```python
from build123d import *

# Parameters (mm, degrees)
SKETCH1_R               = 15.5
BOSS_EXTRUDE1_DEPTH     = 5
CUT_EXTRUDE1_REACH      = 24.483
SKETCH2_R               = 3
CUT_EXTRUDE2_DEPTH      = 23.483327156
CUT_EXTRUDE2_DEPTH_BACK = 23.483327156
SKETCH3_R               = 1.525


with BuildPart() as part:
    # Sketch1 → Boss-Extrude1 (new body)
    with BuildSketch(Plane.XY):
        Circle(SKETCH1_R)
    extrude(amount=BOSS_EXTRUDE1_DEPTH)

    # Sketch2 → Cut-Extrude1 (cut, up to next)
    with BuildSketch(Plane.XY.offset(5), mode=Mode.PRIVATE) as cut_extrude1_sk1:
        Circle(SKETCH2_R)
    cut_extrude1_tool1 = extrude(cut_extrude1_sk1.sketch, amount=-CUT_EXTRUDE1_REACH, mode=Mode.PRIVATE) & part.part
    add(cut_extrude1_tool1.solids().sort_by_distance((0, 0, 5))[0], mode=Mode.SUBTRACT)

    # Sketch3 → Cut-Extrude2 (cut, two sides: drawn at the far end of the back side and taken through both)
    with BuildSketch(Plane.XY.offset(5).offset(-CUT_EXTRUDE2_DEPTH_BACK)):
        with Locations((0, 9)):
            Circle(SKETCH3_R)
        with Locations((7.794228634, -4.5)):
            Circle(SKETCH3_R)
        with Locations((-7.794228634, -4.5)):
            Circle(SKETCH3_R)
    extrude(amount=CUT_EXTRUDE2_DEPTH + CUT_EXTRUDE2_DEPTH_BACK, mode=Mode.SUBTRACT)


solid = part.part
```
Check sheet for the modelled part. Datum: model origin and axes. Units: mm. Round coordinates to 2 decimals unless told otherwise and drop trailing zeros. Write each loop counter-clockwise with the first axis right and the second up, starting at its lowest first coordinate (ties: lowest second). Pieces come first, ordered by that corner, then holes. Notation, with made-up numbers: (64, 35.25) -> (121, 35.25) arc R27 cw to (121, 68.25) -> close; hole circle Ø3 at (-14.75, -31.5). An arc over 180 degrees is marked (long way). One line per question, with ' | ' between items. Start each with the question number.
1. Depth check by flat-ended pin: pin 1 (3 mm diameter, centred on y = -9, z = 1.5, fed in from +X); pin 2 (1 mm diameter, centred on x = 1.5, z = 3.5, fed in from +Y); pin 3 (3 mm diameter, centred on x = 4, z = 2, fed in from -Y). Enter the tip coordinate at first touch or a pass-through.
2. Release check for a two-part mould opening along Y. For faces 1 (the face through (-2.018, 15.368, 2.465)), 2 (the face through (-6.34, -4.04, 2.46)), 3 (the face through (3.2, 0.2, 5)) record: +Y half, -Y half, draft (parallel to the pull), parting line (faces both ways), or undercut.
3. Sectioned sample at D-D, the plane x = 7.5. Record the cut outline in (y, z).
4. Sectioned sample at C-C, the plane y = -4.5. Record the cut outline in (x, z).
5. Sectioned sample at B-B, the plane z = 4.5. Record the cut outline in (x, y) (3 decimals).
6. Scan lines: line 1 along Y through (x, z) = (0, 2.85) (3 decimals); line 2 along X through (y, z) = (-4.5, 1.2); line 3 along X through (y, z) = (-5.5, 0.6). Record each from-to range of solid material in increasing order. Write a range as from..to.
7. Sectioned sample at A-A, the plane x = 0. Record the cut outline in (y, z) (3 decimals).
Taken from the geometry:
1) pin 1: stops at x = 13.56 | pin 2: stops at y = 15.47 | pin 3: stops at y = -15.3
2) face 1: parting line | face 2: undercut | face 3: draft
3) outline: (-13.56, 0) -> (-6, 0) -> (-6, 5) -> (-13.56, 5) -> close; (-3, 0) -> (13.56, 0) -> (13.56, 5) -> (-3, 5) -> close
4) outline: (-14.83, 0) -> (-9.32, 0) -> (-9.32, 5) -> (-14.83, 5) -> close; (-6.27, 0) -> (6.27, 0) -> (6.27, 5) -> (-6.27, 5) -> close; (9.32, 0) -> (14.83, 0) -> (14.83, 5) -> (9.32, 5) -> close
5) outline: circle Ø31 at (0, 0); hole circle Ø3.05 at (-7.794, -4.5); hole circle Ø6 at (0, 0); hole circle Ø3.05 at (0, 9); hole circle Ø3.05 at (7.794, -4.5)
6) line 1: y = -15.5..-3, 3..7.475, 10.525..15.5 | line 2: x = -14.83..-9.32, -6.27..6.27, 9.32..14.83 | line 3: x = -14.49..-8.95, -6.64..6.64, 8.95..14.49
7) outline: (-15.5, 0) -> (-3, 0) -> (-3, 5) -> (-15.5, 5) -> close; (3, 0) -> (7.475, 0) -> (7.475, 5) -> (3, 5) -> close; (10.525, 0) -> (15.5, 0) -> (15.5, 5) -> (10.525, 5) -> close
